```python
from build123d import *

# Parameters (mm, degrees)
ESQUISSE1_W        = 49.2
ESQUISSE1_H        = 25.4
ESQUISSE1_R        = 1.5
BOSS_EXTRU_1_DEPTH = 1.2
CONG_1_R           = 1.5
CONG_2_R           = 1.5
CONG_3_R           = 1.5
CONG_4_R           = 1.5
ESQUISSE3_W        = 13.534356754
ESQUISSE3_H        = 8
BOSS_EXTRU_2_DEPTH = 6.8


with BuildPart() as part:
    # Esquisse1 → Boss.-Extru.1 (new body)
    with BuildSketch(Plane(origin=(0, 0, 0), x_dir=(1, 0, 0), z_dir=(0, 1, 0))):
        Rectangle(ESQUISSE1_W, ESQUISSE1_H)
        with Locations(Location((22.6, 10.7, 0), (0, 0, 270))):
            Circle(ESQUISSE1_R, mode=Mode.SUBTRACT)
        with Locations(Location((22.6, -10.7, 0), (0, 0, 270))):
            Circle(ESQUISSE1_R, mode=Mode.SUBTRACT)
        with Locations(Location((-22.6, -10.7, 0), (0, 0, 270))):
            Circle(ESQUISSE1_R, mode=Mode.SUBTRACT)
        with Locations(Location((-22.6, 10.7, 0), (0, 0, 270))):
            Circle(ESQUISSE1_R, mode=Mode.SUBTRACT)
    extrude(amount=BOSS_EXTRU_1_DEPTH)

    # Congé1
    cong_1_edges = [part.edges().sort_by_distance(p)[0] for p in [
        (24.6, 0.6, 12.7),
    ]]
    fillet(cong_1_edges, radius=CONG_1_R)

    # Congé2
    cong_2_edges = [part.edges().sort_by_distance(p)[0] for p in [
        (-24.6, 0.6, 12.7),
    ]]
    fillet(cong_2_edges, radius=CONG_2_R)

    # Congé3
    cong_3_edges = [part.edges().sort_by_distance(p)[0] for p in [
        (24.6, 0.6, -12.7),
    ]]
    fillet(cong_3_edges, radius=CONG_3_R)

    # Congé4
    cong_4_edges = [part.edges().sort_by_distance(p)[0] for p in [
        (-24.6, 0.6, -12.7),
    ]]
    fillet(cong_4_edges, radius=CONG_4_R)

    # Esquisse3 → Boss.-Extru.2 (add)
    with BuildSketch(Plane(origin=(1.430842634, 1.2, 0.935550953), x_dir=(1, 0, 0), z_dir=(0, 1, 0))):
        with Locations((23.633586999, 0.928816864)):
            Rectangle(ESQUISSE3_W, ESQUISSE3_H)
    extrude(amount=BOSS_EXTRU_2_DEPTH)


solid = part.part
```
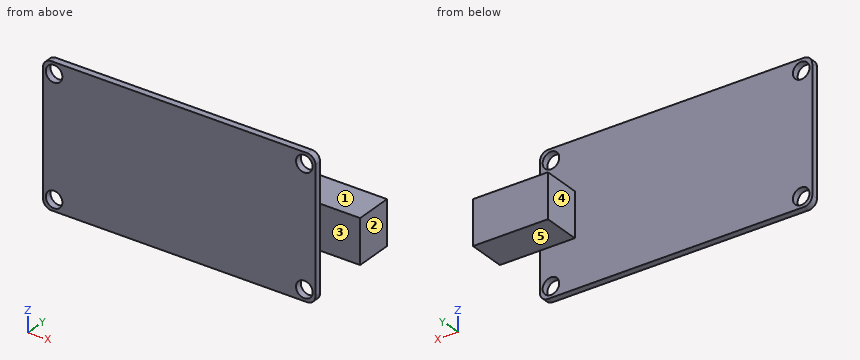
Verification items for the finished model (mm, model axes). Face numbers are marked on the shaded views. A direction names the side the tool comes from. Round coordinates to 2 decimals unless told otherwise and drop trailing zeros. Write each loop counter-clockwise with the first axis right and the second up, starting at its lowest first coordinate (ties: lowest second). Pieces come first, ordered by that corner, then holes. Notation, with made-up numbers: (-38.75, 27.25) - (5.25, 27.25) arc R6 cw to (5.25, 34.25) - close; hole circle Ø5 at (78, 50). An arc over 180 degrees is marked (long way). Answer as a JSON object with one key per item and string values. Group by question number.
Q1. Thickness scan on line 1 (X direction, y = 0.6, z = -10.7); line 2 (X direction, y = 0.5, z = 11.25); line 3 (Y direction, x = -3, z = -2). Record the ranges inside material, lowest first.
Q2. Section check C-C, the plane y = 0.5. Enter the section's corners in (x, z), plus the area to 3 significant figures.
Q3. Section check A-A, the plane x = -22.6. Enter the section's corners in (y, z).
Q4. Go/stop test with flat-tipped pins: pin 1 Ø1.3 at (y, z) = (0.5, -5.5) entering from +X; pin 2 Ø4 at (y, z) = (3.5, 0) entering from -X; pin 3 Ø4 at (x, z) = (-22.6, 10.7) entering from +Y. Record where each tip stops, or that it passes through.
Q5. Section check B-B, the plane z = 10.7. Enter the section's corners in (x, y).
Q6. Tool access check on the marked faces 1, 2, 3, 4 and 5. Record the directions out of +Z, -Z, +X, -X, +Y, -Y that give a thin tool (end or side, any length) a straight path to the whole face; none if there is none.
Q7. Section check D-D, the plane z = 0.5. Enter the section's corners in (x, y).
Found:
{
 "1": {"line 1": "x = -24.6 to -24.1, -21.1 to 21.1, 24.1 to 24.6", "line 2": "x = -24.6 to -24, -21.2 to 21.2, 24 to 24.6", "line 3": "y = 0 to 1.2"},
 "2": {"outline": "(-24.6, -11.2) arc R1.5 ccw to (-23.1, -12.7) - (23.1, -12.7) arc R1.5 ccw to (24.6, -11.2) - (24.6, 11.2) arc R1.5 ccw to (23.1, 12.7) - (-23.1, 12.7) arc R1.5 ccw to (-24.6, 11.2) - close; hole circle Ø3 at (-22.6, -10.7); hole circle Ø3 at (-22.6, 10.7); hole circle Ø3 at (22.6, -10.7); hole circle Ø3 at (22.6, 10.7)", "area": "1,220 mm^2"},
 "3": {"outline": "(0, -12.7) - (1.2, -12.7) - (1.2, -12.2) - (0, -12.2) - close; (0, -9.2) - (1.2, -9.2) - (1.2, 9.2) - (0, 9.2) - close; (0, 12.2) - (1.2, 12.2) - (1.2, 12.7) - (0, 12.7) - close"},
 "4": {"pin 1": "stops at x = 24.6", "pin 2": "stops at x = 18.3", "pin 3": "stops at y = 1.2"},
 "5": {"outline": "(-24.6, 0) - (-24.1, 0) - (-24.1, 1.2) - (-24.6, 1.2) - close; (-21.1, 0) - (21.1, 0) - (21.1, 1.2) - (-21.1, 1.2) - close; (24.1, 0) - (24.6, 0) - (24.6, 1.2) - (24.1, 1.2) - close"},
 "6": {"face 1": "+Z, +X, -X, +Y", "face 2": "+Z, -Z, +X, +Y, -Y", "face 3": "+Z, -Z, +X, -Y", "face 4": "+Z, -Z, -X, +Y", "face 5": "-Z, +X, -X, +Y"},
 "7": {"outline": "(-24.6, 0) - (24.6, 0) - (24.6, 1.2) - (31.83, 1.2) - (31.83, 8) - (18.3, 8) - (18.3, 1.2) - (-24.6, 1.2) - close"}
}
